For this review, take the finished solid that the model builds, in its own axes (mm). A direction names the side the tool comes from. Coordinates: 2 decimals unless noted, no trailing zeros. Order: outer loops, then holes, each group sorted by start corner. A loop starts at its lowest first (then second) coordinate and runs counter-clockwise, first axis right, second up. Notation, with made-up numbers: (-19.5, 74) -> (3.5, 74) arc R24 cw to (3.5, 93) -> close; hole circle Ø4 at (56.5, -18.5). An arc over 180 degrees is marked (long way). Write item = value, one per line. Start each with the question number.
1) Consider section D-D on y = 27.5. Give the boundary of the cut face in (x, z).
2) Insertion check: pin 1 Ø1 at (x, z) = (-4, -19) entering from -Y; pin 2 Ø4 at (x, z) = (-8, -2) entering from +Y; pin 3 Ø12 at (y, z) = (-2, -17) entering from +X; pin 4 Ø13 at (x, z) = (20.88, 19.96) entering from +Y. Each pin has a flat end and moves straight along its axis. Give the tip position at first contact, or say it passes through.
3) Consider section A-A on z = 26. Give the boundary of the cut face in (x, y), and give its area (3 significant figures).
4) Wall thickness on probe 1 along Z at (x, y) = (16.5, 42.5); probe 2 along Z at (x, y) = (17.5, 27.5); probe 3 along Y at (x, z) = (-11, -18): over which ranges is each line inside the solid? List them lowest first. Write a range as [from, to].
5) Draft analysis for pull direction X (two halves, no side actions). For faces 1 (the face through (-26.99, 0.99, 27.15)), 2 (the face through (-27.4, 2, 26.4)), 3 (the face through (0, 2, 0)), state which applies: +X half, -X half, draft (parallel to the pull), parting line (faces both ways), or undercut.
6) Consider section C-C on z = -18. Give the boundary of the cut face in (x, y), and give its area (3 significant figures).
7) Machinability: for faces 4 (the face through (15.616, 34.045, -14.725)), 5 (the face through (-5, -10, 9)), 6 (the face through (29.5, 34.04, 17.62)), 7 (the face through (-6.753, -4.93, 7.647)), which of the approach directions +Z, -Z, +X, -X, +Y, -Y give a long, thin tool a straight path to every point of the face, cutting with its end or side? Answer none if there is none.
8) Consider section B-B on x = -23.5. Give the boundary of the cut face in (y, z), and give its area (3 significant figures).
from build123d import *

# Parameters (mm, degrees)
BOSS_EXTRUDE1_DEPTH  = 2
BOSS_EXTRUDE9_DEPTH  = 65
SKETCH6_R            = 8
CUT_EXTRUDE3_DEPTH   = 78.787752397
SKETCH7_R            = 2
BOSS_EXTRUDE10_DEPTH = 10
SKETCH8_R            = 2
BOSS_EXTRUDE11_DEPTH = 10


with BuildPart() as part:
    # Sketch2 → Boss-Extrude1 (new body)
    with BuildSketch(Plane(origin=(0, 0, 0), x_dir=(1, 0, 0), z_dir=(0, 1, 0))):
        with BuildLine():
            Line((-10, 30), (20, 30))
            ThreePointArc((20, 30), (27.071067812, 27.071067812), (30, 20))
            Line((30, 20), (30, -20))
            ThreePointArc((30, -20), (27.071067812, -27.071067812), (20, -30))
            Line((20, -30), (-20, -30))
            ThreePointArc((-20, -30), (-27.071067812, -27.071067812), (-30, -20))
            Line((-30, -20), (-30, 10))
            ThreePointArc((-30, 10), (-24.142135624, 24.142135624), (-10, 30))
        make_face()
    extrude(amount=BOSS_EXTRUDE1_DEPTH)

    # Sketch5 → Boss-Extrude9 (add)
    with BuildSketch(Plane(origin=(0, 2, 0), x_dir=(1, 0, 0), z_dir=(0, 1, 0))):
        with BuildLine():
            Line((-30.116404199, -19.68082931), (-28.263425554, -20.100912803))
            ThreePointArc((-28.263425554, -20.100912803), (-15.988853518, -15.236719498), (-15.896791782, -28.439636592))
            Line((-15.896791782, -28.439636592), (-14.812694906, -30))
            ThreePointArc((-14.812694906, -30), (-14.926621305, -13.661390096), (-30.116404199, -19.68082931))
        make_face()
        with BuildLine():
            Line((20.977105182, -29.863851609), (20.875608793, -27.964371901))
            ThreePointArc((20.875608793, -27.964371901), (14.520196839, -15.105489427), (28.595658733, -17.866556627))
            Line((28.595658733, -17.866556627), (30.429170594, -17.368325499))
            ThreePointArc((30.429170594, -17.368325499), (12.980066991, -13.991900081), (20.977105182, -29.863851609))
        make_face()
        with BuildLine():
            Line((13.764397277, 30), (16.80629322, 30))
            ThreePointArc((16.80629322, 30), (17.733969491, 15.754964907), (28.664900588, 24.936269467))
            Line((28.664900588, 24.936269467), (29.994544588, 19.258061402))
            ThreePointArc((29.994544588, 19.258061402), (15.411631267, 14.856680059), (13.764397277, 30))
        make_face()
    extrude(amount=BOSS_EXTRUDE9_DEPTH)

    # Sketch6 → Cut-Extrude3 (cut, through all)
    with BuildSketch(Plane(origin=(0, 2, 0), x_dir=(1, 0, 0), z_dir=(0, 1, 0))):
        with Locations((20.875608793, 23.112281164)):
            Circle(SKETCH6_R)
        with Locations(Location((-20.461410206, -21.869685402, 0), (0, 0, 167.226551727))):
            Circle(SKETCH6_R)
        with Locations(Location((20.875608793, -19.964371901, 0), (0, 0, 270))):
            Circle(SKETCH6_R)
    extrude(amount=-CUT_EXTRUDE3_DEPTH, mode=Mode.SUBTRACT)

    # Sketch7 → Boss-Extrude10 (add)
    with BuildSketch(Plane.XZ):
        with Locations(Location((6.600213653, -6.067854065, 0), (0, 0, 90))):
            Circle(SKETCH7_R)
    extrude(amount=BOSS_EXTRUDE10_DEPTH)

    # Sketch8 → Boss-Extrude11 (add)
    with BuildSketch(Plane.XZ):
        with Locations(Location((-5.40151955, 9.120930292, 0), (0, 0, 90))):
            Circle(SKETCH8_R)
    extrude(amount=BOSS_EXTRUDE11_DEPTH)


solid = part.part
Answer sheet:
q1.outline = (-30.12, 19.68) arc R9.9 ccw (long way) to (-14.81, 30) -> (-15.9, 28.44) arc R8 cw (long way) to (-28.26, 20.1) -> close; (13.76, -30) -> (16.81, -30) arc R8 cw (long way) to (28.66, -24.94) -> (29.99, -19.26) arc R9.9 ccw (long way) to start; (20.88, 27.96) -> (20.98, 29.86) arc R9.9 ccw (long way) to (30.43, 17.37) -> (28.6, 17.87) arc R8 cw (long way) to start
q2.pin_1 = 0
q2.pin_2 = 2
q2.pin_3 = 30
q2.pin_4 = through
q3.outline = (-28, 0) -> (-27.31, 0) -> (-27.31, 2) -> (-28, 2) -> close; (-13.61, 0) -> (15.62, 0) -> (15.62, 67) -> (13.03, 67) -> (13.03, 2) -> (-11.46, 2) -> (-11.46, 67) -> (-13.61, 67) -> close; (26.13, 0) -> (28, 0) -> (28, 2) -> (26.13, 2) -> close
q3.area = 372 mm2
q4.probe_1 = [-30, -29.81], [-16.41, -14.23], [11.08, 13.27], [26.66, 28.84]
q4.probe_2 = [-15.86, -13.81], [10.66, 12.71], [27.22, 29.27]
q4.probe_3 = [0, 2]
q5.face_1 = -X half
q5.face_2 = draft
q5.face_3 = undercut
q6.outline = (-28.33, 0) -> (14.72, 0) -> (14.72, 67) -> (12.4, 67) -> (12.4, 2) -> (-28.33, 2) -> close; (27.03, 0) -> (30, 0) -> (30, 2) -> (29.35, 2) -> (29.35, 67) -> (27.03, 67) -> close
q6.area = 394 mm2
q7.face_4 = +Y
q7.face_5 = +Z, -Z, +X, -X, -Y
q7.face_6 = +Z, +X, +Y
q7.face_7 = -Y
q8.outline = (0, -24.76) -> (2, -24.76) -> (2, 12.45) -> (67, 12.45) -> (67, 14.47) -> (0, 14.47) -> close; (0, 29.27) -> (2, 29.27) -> (2, 29.37) -> (0, 29.37) -> close
q8.area = 210 mm2
